Here's how the part is built. I have some questions about the finished solid (model axes, mm). Give positions to 0.01 mm unless a question says otherwise; leave off trailing zeros. Order: outer loops, then holes, each group sorted by start corner. A loop starts at its lowest first (then second) coordinate and runs counter-clockwise, first axis right, second up. Notation, with made-up numbers: M 79,1 L 113,1 A36 cw 113,35 Z; hole C 66.25,57.5 d6. An arc over 180 degrees is marked long. Use one line per item in the form item = value.
from build123d import *

# Parameters (mm, degrees)
BOSS_EXTRUDE1_DEPTH = 5
FILLET1_R           = 3


with BuildPart() as part:
    # Sketch1 → Boss-Extrude1 (new body)
    with BuildSketch(Plane(origin=(0, 0, 0), x_dir=(1, 0, 0), z_dir=(0, 1, 0))):
        Polygon((-30.200218536, 0), (-15.100109268, -26.154156452), (15.100109268, -26.154156452), (30.200218536, 0), (15.100109268, 26.154156452), (-15.100109268, 26.154156452), align=None)
    extrude(amount=BOSS_EXTRUDE1_DEPTH)

    # Fillet1
    fillet1_edges = [part.edges().sort_by_distance(p)[0] for p in [
        (-15.100109268, 2.5, -26.154156452),
        (15.100109268, 2.5, -26.154156452),
        (30.200218536, 2.5, 0),
        (15.100109268, 2.5, 26.154156452),
        (-15.100109268, 2.5, 26.154156452),
        (-30.200218536, 2.5, 0),
    ]]
    fillet(fillet1_edges, radius=FILLET1_R)


solid = part.part
Q1. I want a section at B-B on z = -8. Write out the boundary of the cut face in (x, y), then the cut area to 3 significant figures.
Found:
outline = M -25.58,0 L 25.58,0 L 25.58,5 L -25.58,5 Z
area = 256 mm²
Q2. I want a section at A-A on y = 0.9. Write out the boundary of the cut face in (x, z).
Found:
outline = M -29.33,-1.5 L -15.97,-24.65 A3 ccw -13.37,-26.15 L 13.37,-26.15 A3 ccw 15.97,-24.65 L 29.33,-1.5 A3 ccw 29.33,1.5 L 15.97,24.65 A3 ccw 13.37,26.15 L -13.37,26.15 A3 ccw -15.97,24.65 L -29.33,1.5 A3 ccw Z
Q3. I want a section at C-C on x = -18.5. Write out the boundary of the cut face in (y, z).
Found:
outline = M 0,-20.27 L 5,-20.27 L 5,20.27 L 0,20.27 Z
Q4. I need wall thicknesses on L1, parallel to X at y = 2.4, z = -11.5; L2, parallel to X at y = 1.4, z = -20; L3, parallel to Z at x = -25, y = 1.55. Which ranges of each line are inside material? Lowest first, please.
Found:
L1 = -23.56 to 23.56
L2 = -18.65 to 18.65
L3 = -9.01 to 9.01
Q5. I'm going to push a flat-ended pin straight in: pin 1 Ø2 at (x, z) = (-1, 2) entering from -Y. Where does the tip first touch, or does it pass through?
Found:
pin_1 = 0
